Job drawing, mm, ordinate dimensions from the low corner. One solid piece. A direction names the side the tool comes from. Give positions to 0.01 mm unless a question says otherwise; leave off trailing zeros. Loops run counter-clockwise (first coordinate to the right, second up) from the corner with the lowest first, then second, coordinate; pieces in that order, holes last. Notation, with made-up numbers: (-1, 79) -> (14, 79) arc R27 cw to (14, 113) -> close; hole circle Ø10 at (9, -21). An arc over 180 degrees is marked (long way). Answer as a JSON object with one key per item and string values. Group by question number.
Q1. Band-saw the part on D-D, the plane x = 5.75. Write the cut outline in (y, z) (1 decimal), plus the area to 3 significant figures.
Q2. Band-saw the part on C-C, the plane x = 10. Write the cut outline in (y, z).
Q3. Tool access for the marked faces 1 and 2: list every direction of +Z, -Z, +X, -X, +Y, -Y with a clear straight run to the whole face (end or side of a thin tool).
Q4. Wall check: probe 1 along Y at (x, z) = (10, 1.65); probe 2 along Z at (x, y) = (18, 10.5); probe 3 along Y at (x, z) = (10, 0.9). Give the ranges that are in metal, low to high. Write a range as from..to.
Q5. Band-saw the part on A-A, the plane z = 0.45. Write the cut outline in (x, y) (1 decimal), plus the area to 3 significant figures.
Q6. Drop a flat-ended pin along its axis: pin 1 (1 mm diameter, centred on x = 5, z = 2, fed in from +Y) (1 decimal). Give the stop position or say it passes through.
Q7. Two-plate mould, pull along X, no slides. Class the marked faces 3, 4 and 5: pulls with the +X half, pulls with the -X half, needs draft (parallel to the pull), parting line crosses it, or undercut.
Q8. Band-saw the part on B-B, the plane y = 6. Write the cut outline in (x, z) (1 decimal).
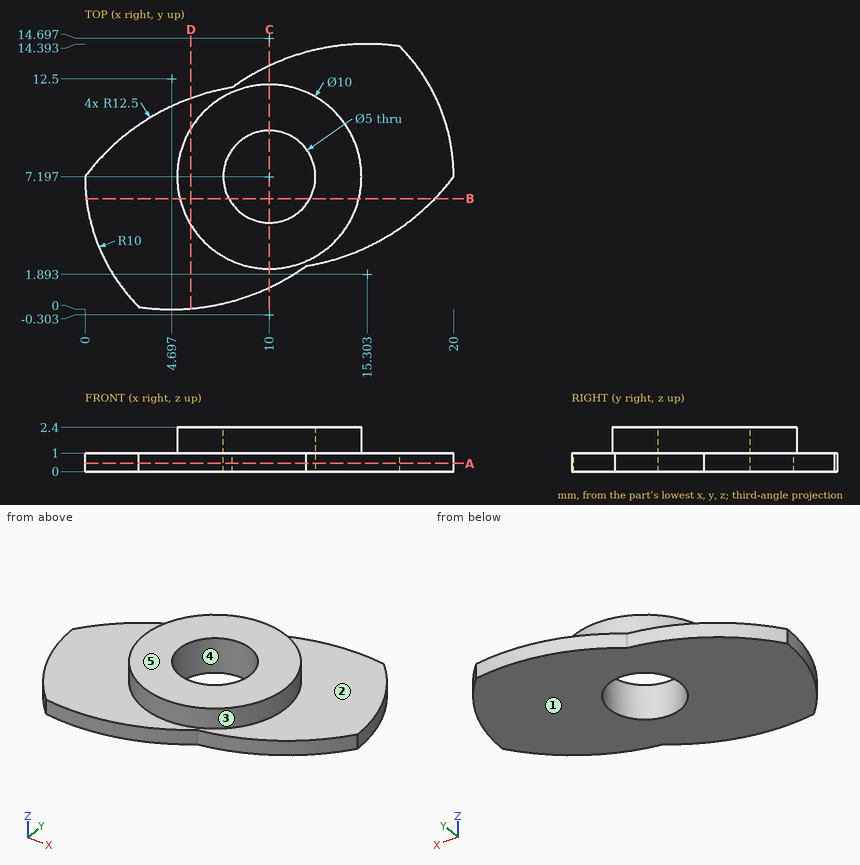
Worked answers:
{
 "1": {"outline": "(0, 0) -> (11.5, 0) -> (11.5, 1) -> (9.8, 1) -> (9.8, 2.4) -> (4.6, 2.4) -> (4.6, 1) -> (0, 1) -> close", "area": "18.8 mm2"},
 "2": {"outline": "(1.18, 0) -> (4.7, 0) -> (4.7, 2.4) -> (2.2, 2.4) -> (2.2, 1) -> (1.18, 1) -> close; (9.7, 0) -> (13.21, 0) -> (13.21, 1) -> (12.2, 1) -> (12.2, 2.4) -> (9.7, 2.4) -> close"},
 "3": {"face 1": "-Z, +X, -X, +Y, -Y", "face 2": "+Z"},
 "4": {"probe 1": "2.2..4.7, 9.7..12.2", "probe 2": "0..1", "probe 3": "1.18..4.7, 9.7..13.21"},
 "5": {"outline": "(0, 7.2) arc R10 ccw to (2.9, 0.1) arc R12.5 ccw to (12, 2.4) arc R12.5 ccw to (20, 7.2) arc R10 ccw to (17.1, 14.3) arc R12.5 ccw to (8, 12) arc R12.5 ccw to start; hole circle Ø5 at (10, 7.2)", "area": "178 mm2"},
 "6": {"pin 1": "y = 9.4"},
 "7": {"face 3": "parting line crosses it", "face 4": "undercut", "face 5": "needs draft"},
 "8": {"outline": "(0.1, 0) -> (7.8, 0) -> (7.8, 2.4) -> (5.1, 2.4) -> (5.1, 1) -> (0.1, 1) -> close; (12.2, 0) -> (19, 0) -> (19, 1) -> (14.9, 1) -> (14.9, 2.4) -> (12.2, 2.4) -> close"}
}
